```python
from build123d import *

# Parameters (mm, degrees)
F2_R     = 1
F3_DEPTH = 7


with BuildPart() as f1:
    # F0 (on Front) → F1 (revolve)
    with BuildSketch(Plane.XZ):
        Polygon((2, 123.75), (0, 123.75), (0, 0), (12.5, 0), (12.5, 12), (15, 12), (15, 76), (16, 76), (16, 112), (9.5, 112), (9.5, 113.75), (2, 113.75), align=None)
    revolve(axis=Axis((0, 0, 70.364535), (0, 0, 1)))

    # F2 (on face) → F3 (cut)
    with BuildSketch(Plane.XY.offset(112)):
        with Locations((0, 13)):
            Circle(F2_R)
        with Locations((13, 0)):
            Circle(F2_R)
        with Locations((-13, 0)):
            Circle(F2_R)
        with Locations((0, -13)):
            Circle(F2_R)
    extrude(amount=-F3_DEPTH, mode=Mode.SUBTRACT)


solid = f1.part
```
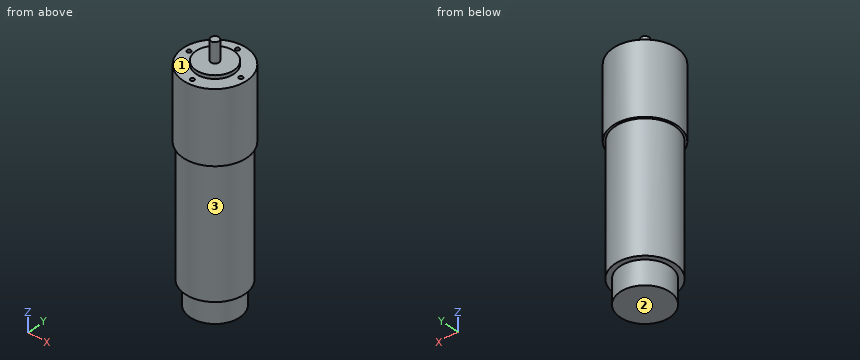
Verification items for the finished model (mm, model axes). Face numbers are marked on the shaded views. A direction names the side the tool comes from. Coordinates: 2 decimals unless noted, no trailing zeros. Write each loop counter-clockwise with the first axis right and the second up, starting at its lowest first coordinate (ties: lowest second). Pieces come first, ordered by that corner, then holes. Notation, with made-up numbers: (80.25, -1.5) - (104.25, -1.5) arc R26 ccw to (104.25, 29.5) - close; hole circle Ø6 at (2.5, 11). An arc over 180 degrees is marked (long way). Write item = value, one per line.
Q1. Go/stop test with flat-tipped pins: pin 1 Ø3 at (x, y) = (-6, -5.5) entering from +Z; pin 2 Ø3 at (x, z) = (12, 46.5) entering from +Y; pin 3 Ø4 at (x, z) = (-11.5, 36) entering from +Y. Record where each tip stops, or that it passes through.
Answer:
pin_1 = 113.75
pin_2 = 10.71
pin_3 = 11.61
Q2. Cross-section at B-B (x = -3.5). Enter the section's corners in (y, z), plus the area to 3 significant figures.
Answer:
outline = (-15.61, 76) - (-14.59, 76) - (-14.59, 12) - (-12, 12) - (-12, 0) - (12, 0) - (12, 12) - (14.59, 12) - (14.59, 76) - (15.61, 76) - (15.61, 112) - (8.83, 112) - (8.83, 113.75) - (-8.83, 113.75) - (-8.83, 112) - (-15.61, 112) - close
area = 3,310 mm²
Q3. Cross-section at C-C (y = 5.5). Enter the section's corners in (x, z), plus the area to 3 significant figures.
Answer:
outline = (-15.02, 76) - (-13.96, 76) - (-13.96, 12) - (-11.22, 12) - (-11.22, 0) - (11.22, 0) - (11.22, 12) - (13.96, 12) - (13.96, 76) - (15.02, 76) - (15.02, 112) - (7.75, 112) - (7.75, 113.75) - (-7.75, 113.75) - (-7.75, 112) - (-15.02, 112) - close
area = 3,160 mm²
Q4. Access from +Z, -Z, +X, -X, +Y, -Y to the whole of each face (thin tool, end or side, straight path). Record for the marked faces 1, 2 and 3.
Answer:
face_1 = +Z
face_2 = -Z, +X, -X, +Y, -Y
face_3 = -Z
Q5. Cross-section at D-D (z = 38). Enter the section's corners in (x, y), plus the area to 3 significant figures.
Answer:
outline = circle Ø30 at (0, 0)
area = 707 mm²
Q6. Material ranges on L1, parallel to Y at x = 0, z = 107.5; L2, parallel to Z at x = -6, y = -14; L3, parallel to Z at x = 12, y = 4.5, recorded low to high. Write a range as from..to.
Answer:
L1 = -16..-14, -12..12, 14..16
L2 = 76..112
L3 = 12..112
Q7. Cross-section at A-A (z = 79). Enter the section's corners in (x, y), plus the area to 3 significant figures.
Answer:
outline = circle Ø32 at (0, 0)
area = 804 mm²
